Read the model definition and answer for the solid it produces. Units are mm, in the model's axes. A direction names the side the tool comes from. Coordinates: 2 decimals unless noted, no trailing zeros. Write each loop counter-clockwise with the first axis right and the second up, starting at its lowest first coordinate (ties: lowest second). Pieces come first, ordered by that corner, then holes.
Item 1: Section A-A (x = -2.5) is taken. Give the vertices of the cut face in (y, z).
Item 2: A tool of negligible diameter and unlimited length cuts with its end or side. For faces 4 (the face through (-2, -2, 0)), 5 (the face through (1, 1, 5)), from which of +Z, -Z, +X, -X, +Y, -Y can it reach the whole face along a straight path? Write none if from no direction.
Item 3: Section C-C (x = -5.5) is taken. Give the vertices of the cut face in (y, z), then the cut area to 3 significant figures.
Item 4: Section D-D (z = 2) is taken. Give the vertices of the cut face in (x, y), then the cut area to 3 significant figures.
Item 5: Section B-B (y = -6.25) is taken. Give the vertices of the cut face in (x, z).
Item 6: Each of these flat-tipped pins is pushed along its axis until it touches: P1, Ø6, axis at x = 6, y = 12, coming from the -Z side; P2, Ø1, axis at y = -1, z = -7.5, coming from the -X side; P3, Ø6, axis at y = 4, z = -10.5, coming from the -X side. Where does it stop, or does it pass through?
Item 7: Determine the mould class of faces 1 (the face through (-12.1, 5.9, 2.5)), 2 (the face through (-1.034, -0.563, -6.648)), 3 (the face through (0.9, -1, -7.4)) for opening direction Y: released by +Y, released by -Y, zero draft, split by the parting line, or undercut.
Item 8: Straight lines are drawn through the part: probe 1 along X at (y, z) = (4.25, 1); probe 2 along Z at (x, y) = (9.25, -3.5); probe 3 along Y at (x, z) = (-4, -9.75). For each, find the intervals that lie inside material, in ascending order.
from build123d import *

# Parameters (mm, degrees)
SKETCH_1_R          = 15
SKETCH_1_R_2        = 1.6
EXTRUDE_1_DEPTH     = 5
SKETCH_2_R          = 6
EXTRUDE_2_DEPTH     = 15
SKETCH_3_R          = 4.1
CUT_EXTRUDE_1_DEPTH = 21
SKETCH_4_R          = 1.6
CUT_EXTRUDE_2_DEPTH = 15


with BuildPart() as part:
    # 草图1 → 凸台-拉伸1 (new body)
    with BuildSketch(Plane.XY):
        with Locations((-1.893979513, 4.311637078)):
            Circle(SKETCH_1_R)
        with Locations((-1.893979513, 14.311637078)):
            Circle(SKETCH_1_R_2, mode=Mode.SUBTRACT)
        with Locations((8.106020487, 4.311637078)):
            Circle(SKETCH_1_R_2, mode=Mode.SUBTRACT)
        with Locations((-1.893979513, -5.688362922)):
            Circle(SKETCH_1_R_2, mode=Mode.SUBTRACT)
        with Locations((-11.893979513, 4.311637078)):
            Circle(SKETCH_1_R_2, mode=Mode.SUBTRACT)
    extrude(amount=EXTRUDE_1_DEPTH)

    # 草图2 → 凸台-拉伸2 (add)
    with BuildSketch(Plane.XY):
        with Locations((-1.893979513, 4.311637078)):
            Circle(SKETCH_2_R)
    extrude(amount=-EXTRUDE_2_DEPTH)

    # 草图3 → 切除-拉伸1 (cut, through all)
    with BuildSketch(Plane(origin=(0, 0, -15), x_dir=(-1, 0, 0), z_dir=(0, 0, -1))):
        with Locations((1.893979513, 4.311637078)):
            Circle(SKETCH_3_R)
    extrude(amount=-CUT_EXTRUDE_1_DEPTH, mode=Mode.SUBTRACT)

    # 草图4 → 切除-拉伸2 (cut, symmetric)
    with BuildSketch(Plane(origin=(0, 0, 0), x_dir=(1, 0, 0), z_dir=(0, 1, 0))):
        with Locations((-1.893979513, 5.299041656)):
            Circle(SKETCH_4_R)
    extrude(amount=CUT_EXTRUDE_2_DEPTH, both=True, mode=Mode.SUBTRACT)


solid = part.part
Established:
1. outline: (-10.68, 0) - (-7.17, 0) - (-7.17, 5) - (-10.68, 5) - close; (-4.21, 0) - (-1.66, 0) - (-1.66, -3.82) - (0.26, -3.82) - (0.26, 5) - (-4.21, 5) - close; (-1.66, -15) - (0.26, -15) - (0.26, -6.78) - (-1.66, -6.78) - close; (8.37, -15) - (10.28, -15) - (10.28, -6.78) - (8.37, -6.78) - close; (8.37, -3.82) - (10.28, -3.82) - (10.28, 0) - (12.83, 0) - (12.83, 5) - (8.37, 5) - close; (15.79, 0) - (19.3, 0) - (19.3, 5) - (15.79, 5) - close
2. face 4: -Z
2. face 5: +Z, +X, -X, +Y, -Y
3. outline: (-10.25, 0) - (-0.48, 0) - (-0.48, -15) - (2.36, -15) - (2.36, 5) - (-10.25, 5) - close; (6.26, -15) - (9.11, -15) - (9.11, 0) - (18.87, 0) - (18.87, 5) - (6.26, 5) - close
3. area: 211 mm2
4. outline: circle Ø30 at (-1.89, 4.31); hole circle Ø3.2 at (-11.89, 4.31); hole circle Ø8.2 at (-1.89, 4.31); hole circle Ø3.2 at (-1.89, -5.69); hole circle Ø3.2 at (-1.89, 14.31); hole circle Ø3.2 at (8.11, 4.31)
4. area: 622 mm2
5. outline: (-12.55, 0) - (-3.39, 0) - (-3.39, 5) - (-12.55, 5) - close; (-0.4, 0) - (8.76, 0) - (8.76, 5) - (-0.4, 5) - close
6. P1: stops at z = 0
6. P2: stops at x = -5.48
6. P3: stops at x = -7.89
7. face 1: undercut
7. face 2: zero draft
7. face 3: split by the parting line
8. probe 1: x = -16.89 to -13.49, -10.3 to -5.99, 2.21 to 6.51, 9.7 to 13.11
8. probe 2: z = 0 to 5
8. probe 3: y = -1.31 to 0.79, 7.83 to 9.93
